Autodesk Inventor part; units mm, degrees
ref_plane "YZ Plane" through (0, 0, 0) normal (1, 0, 0) x (0, 1, 0)
ref_plane "XZ Plane" through (0, 0, 0) normal (0, 1, 0) x (-1, 0, 0)
ref_plane "XY Plane" through (0, 0, 0) normal (0, 0, 1) x (1, 0, 0)
sketch "Sketch1" plane through (0, 0, 0) normal (0, 1, 0) x (-1, 0, 0)
  line L0 (0, 0) -> (0, -4.5)
  line L1 (0, 0) -> (23, 0)
  line L2 (23, 0) -> (23, -23)
  line L3 (23, -23) -> (18.5, -23)
  line L4 (0, -4.5) -> (18.5, -4.5)
  line L5 (18.5, -4.5) -> (18.5, -23)
  dimension "d0" = 4.5
  dimension "d1" = 23
  dimension "d2" = 23
  dimension "d3" = 4.5
extrude "Extrusion1" add sketch "Sketch1" along normal blind 23
fillet "Fillet1" radius 2 4 edges at (-20.75, 23, -23) (-20.75, 0, -23) (0, 0, -2.25) (0, 23, -2.25)
sketch "Sketch2" plane through (-18.5, 0, -4.5) normal (0, 0, -1) x (-1, 0, 0)
  circle A0 centre (-14.5, 19) radius 2
  circle A1 centre (-4.5, 19) radius 2
  circle A2 centre (-4.5, 4) radius 2
  circle A3 centre (-14.5, 4) radius 2
  line L0 (-16.5, 23) -> (0, 23)
  line L1 (-16.5, 0) -> (0, 0)
  line L2 (-18.5, 2) -> (-18.5, 21)
  line L3 (4.5, 2) -> (4.5, 21)
  point P0 (-18.5, 0)
  dimension "d7" = 4
  dimension "d8" = 4
  dimension "d9" = 4
  dimension "d10" = 4
  dimension "d11" = 4
  dimension "d12" = 15
  dimension "d13" = 4
  dimension "d14" = 4
  dimension "d15" = 10
  dimension "d16" = 4
  dimension "d17" = 4
  dimension "d18" = 9
  dimension "d19" = 9
hole "Hole1" at (-4, 19, -4.5) at (-4, 4, -4.5) at (-14, 19, -4.5) at (-14, 4, -4.5) direction (0, 0, 1) diameter 4 depth 4.5 tip angle 118
sketch "Sketch3" plane through (-18.5, 0, -4.5) normal (1, 0, 0) x (0, 0, -1)
  line L0 (4, 16.5) -> (14, 16.5) construction
  line L1 (14, 16.5) -> (14, 6.5) construction
  line L2 (14, 6.5) -> (4, 6.5) construction
  line L3 (4, 6.5) -> (4, 16.5) construction
  circle A0 centre (4, 16.5) radius 2
  circle A1 centre (14, 16.5) radius 2
  circle A2 centre (14, 6.5) radius 2
  circle A3 centre (4, 6.5) radius 2
  line L4 (0, 23) -> (16.5, 23)
  line L5 (-4.5, 2) -> (-4.5, 21)
  line L6 (18.5, 2) -> (18.5, 21)
  point P0 (-4.5, 0)
  dimension "d27" = 4
  dimension "d28" = 4
  dimension "d29" = 4
  dimension "d30" = 4
  dimension "d31" = 6.5
  dimension "d32" = 10
  dimension "d33" = 10
  dimension "d34" = 8.5
  dimension "d35" = 4.5
hole "Hole2" at (-18.5, 16.5, -8.5) at (-18.5, 16.5, -18.5) at (-18.5, 6.5, -8.5) at (-18.5, 6.5, -18.5) direction (-1, 0, 0) diameter 4 depth 4.5 tip angle 118
chamfer "Chamfer1" distance 0.25 angle 45 28 edges at (-10.25, 23, -4.5) (-0.5858, 22.4142, -4.5) (0, 11.5, -4.5) (-0.5858, 0.5858, -4.5) (-10.25, 0, -4.5) (-12.5, 23, 0) (-0.5858, 22.4142, 0) (0, 11.5, 0) (-0.5858, 0.5858, 0) (-12.5, 0, 0) (-18.5, 23, -12.75) (-18.5, 22.4142, -22.4142) (-18.5, 11.5, -23) (-18.5, 0.5858, -22.4142) (-18.5, 0, -12.75) (-23, 23, -10.5) (-23, 22.4142, -22.4142) (-23, 11.5, -23) (-23, 0.5858, -22.4142) (-23, 0, -10.5) (-18.5, 16.5, -6.5) (-18.5, 16.5, -16.5) (-18.5, 6.5, -6.5) (-18.5, 6.5, -16.5) (-14, 17, -4.5) (-4, 17, -4.5) (-14, 2, -4.5) (-4, 2, -4.5)
properties part number "HUDSON-1-06 FRONT BUFFER BEAM ANGLE"
Verification items for the finished model (mm, model axes). Round coordinates to 2 decimals unless told otherwise and drop trailing zeros. Loops run counter-clockwise (first coordinate to the right, second up) from the corner with the lowest first, then second, coordinate; pieces in that order, holes last. Notation, with made-up numbers: (-15.75, -16) - (35.25, -16) arc R5 cw to (35.25, -12) - close; hole circle Ø11 at (-19.75, -18). An arc over 180 degrees is marked (long way). Use a Markdown table: item, result. Add a question column.
1. Thickness scan on probe 1 along Y at (x, z) = (-4, -2.7); probe 2 along X at (y, z) = (4, -0.95); probe 3 along Z at (x, y) = (-21.7, 6.5). Record the ranges inside material, lowest first. Write a range as [from, to].
2. Section check A-A, the plane z = -8.5. Record the boundary of the cut face in (x, y), plus the area to 4 significant figures.
3. Gauge pin test, flat ends, axial feed: pin 1 (3 mm diameter, centred on x = -14, y = 4, fed in from +Z); pin 2 (6 mm diameter, centred on x = -6.5, y = 16.5, fed in from +Z); pin 3 (6.5 mm diameter, centred on y = 6.5, z = -18.5, fed in from +X); pin 4 (5 mm diameter, centred on x = -4, y = 19, fed in from -Z). Record the tip position at first contact, or that the pin passes through.
4. Section check B-B, the plane x = -19.25. Record the boundary of the cut face in (y, z), plus the area to 3 significant figures.
5. Release check for a two-part mould opening along X. For faces 1 (the face through (-18.627, 22.342, -22.312)), 2 (the face through (-20.72, 22.4, -22.43)), 3 (the face through (-22.873, 0.658, -22.312)), 4 (the face through (-2.8, 17.4, -2.1)) record: released by +X, released by -X, zero draft, split by the parting line, or undercut.
6. Section check D-D, the plane y = 10. Record the boundary of the cut face in (x, z), plus the area to 3 significant figures.
7. Section check C-C, the plane x = -4. Record the boundary of the cut face in (y, z).
Checks:
| question | item | result |
|---|---|---|
| 1 | probe 1 | y = [0, 2], [6, 17], [21, 23] |
| 1 | probe 2 | x = [-23, -16], [-12, -6], [-2, 0] |
| 1 | probe 3 | z = [-23, -20.5], [-16.5, -10.5], [-6.5, 0] |
| 2 | outline | (-23, 0.25) - (-22.75, 0) - (-18.75, 0) - (-18.5, 0.25) - (-18.5, 4.25) - (-18.75, 4.5) - (-23, 4.5) - close; (-23, 8.5) - (-18.75, 8.5) - (-18.5, 8.75) - (-18.5, 14.25) - (-18.75, 14.5) - (-23, 14.5) - close; (-23, 18.5) - (-18.75, 18.5) - (-18.5, 18.75) - (-18.5, 22.75) - (-18.75, 23) - (-22.75, 23) - (-23, 22.75) - close |
| 2 | area | 67.25 mm^2 |
| 3 | pin 1 | passes through |
| 3 | pin 2 | stops at z = 0 |
| 3 | pin 3 | stops at x = -18.5 |
| 3 | pin 4 | stops at z = -4.5 |
| 4 | outline | (0, -21) arc R2 ccw to (2, -23) - (21, -23) arc R2 ccw to (23, -21) - (23, -0.25) - (22.75, 0) - (0.25, 0) - (0, -0.25) - close; hole circle Ø4 at (6.5, -18.5); hole circle Ø4 at (6.5, -8.5); hole circle Ø4 at (16.5, -18.5); hole circle Ø4 at (16.5, -8.5) |
| 4 | area | 477 mm^2 |
| 5 | face 1 | released by +X |
| 5 | face 2 | zero draft |
| 5 | face 3 | released by -X |
| 5 | face 4 | undercut |
| 6 | outline | (-23, -22.75) - (-22.75, -23) - (-18.75, -23) - (-18.5, -22.75) - (-18.5, -4.5) - (-0.25, -4.5) - (0, -4.25) - (0, -0.25) - (-0.25, 0) - (-23, 0) - close |
| 6 | area | 187 mm^2 |
| 7 | outline | (0, -4.25) - (0.25, -4.5) - (1.75, -4.5) - (2, -4.25) - (2, 0) - (0.25, 0) - (0, -0.25) - close; (6, -4.25) - (6.25, -4.5) - (16.75, -4.5) - (17, -4.25) - (17, 0) - (6, 0) - close; (21, -4.25) - (21.25, -4.5) - (22.75, -4.5) - (23, -4.25) - (23, -0.25) - (22.75, 0) - (21, 0) - close |
